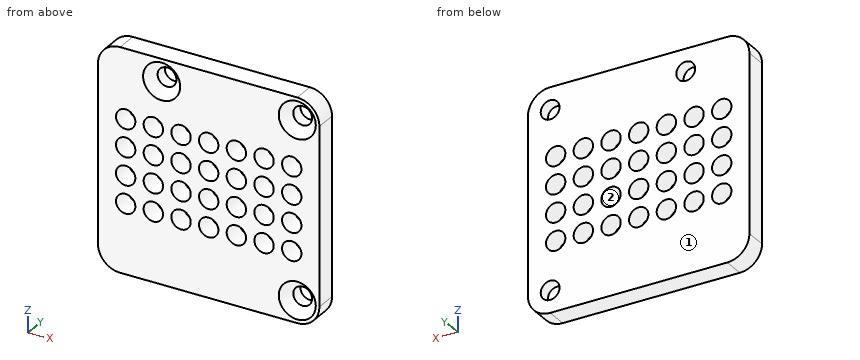
```python
from build123d import *

# Parameters (mm, degrees)
SKETCH1_R                                           = 1.6
BOSS_EXTRUDE1_DEPTH                                 = 3.85
CSK_FOR_M3_COUNTERSUNK_FLAT_HEAD_SCREW1_D           = 3.4
CSK_FOR_M3_COUNTERSUNK_FLAT_HEAD_SCREW1_CSINK_D     = 6.7
CSK_FOR_M3_COUNTERSUNK_FLAT_HEAD_SCREW1_CSINK_ANGLE = 90
SKETCH4_R                                           = 1.75
CUT_EXTRUDE1_DEPTH                                  = 12.5


with BuildPart() as part:
    # Sketch1 → Boss-Extrude1 (new body)
    with BuildSketch(Plane(origin=(0, 0, 0), x_dir=(1, 0, 0), z_dir=(0, 1, 0))):
        with BuildLine():
            Line((4, 0), (36, 0))
            ThreePointArc((36, 0), (38.828427125, 1.171572875), (40, 4))
            Line((40, 4), (40, 36))
            ThreePointArc((40, 36), (38.828427125, 38.828427125), (36, 40))
            Line((36, 40), (4, 40))
            ThreePointArc((4, 40), (1.171572875, 38.828427125), (0, 36))
            Line((0, 36), (0, 4))
            ThreePointArc((0, 4), (1.171572875, 1.171572875), (4, 0))
        make_face()
        with Locations(Location((11.5, 4, 0), (0, 0, 90))):
            Circle(SKETCH1_R, mode=Mode.SUBTRACT)
        with Locations(Location((36, 4, 0), (0, 0, 90))):
            Circle(SKETCH1_R, mode=Mode.SUBTRACT)
        with Locations(Location((36, 36, 0), (0, 0, 90))):
            Circle(SKETCH1_R, mode=Mode.SUBTRACT)
    extrude(amount=BOSS_EXTRUDE1_DEPTH)

    # CSK for M3 Countersunk Flat Head Screw1 (through all)
    with Locations(Plane(origin=(0, 0, 0), x_dir=(-1, 0, 0), z_dir=(0, -1, 0))):
        with Locations((-11.5, 4), (-36, 4), (-36, 36)):
            CounterSinkHole(CSK_FOR_M3_COUNTERSUNK_FLAT_HEAD_SCREW1_D / 2, CSK_FOR_M3_COUNTERSUNK_FLAT_HEAD_SCREW1_CSINK_D / 2, counter_sink_angle=CSK_FOR_M3_COUNTERSUNK_FLAT_HEAD_SCREW1_CSINK_ANGLE)

    # Sketch4 → Cut-Extrude1 (cut)
    with BuildSketch(Plane(origin=(0, 3.85, 0), x_dir=(1, 0, 0), z_dir=(0, 1, 0))):
        with Locations(Location((5, 22.5, 0), (0, 0, 270))):
            Circle(SKETCH4_R)
        with Locations(Location((10, 22.5, 0), (0, 0, 270))):
            Circle(SKETCH4_R)
        with Locations(Location((5, 17.5, 0), (0, 0, 270))):
            Circle(SKETCH4_R)
        with Locations(Location((10, 17.5, 0), (0, 0, 270))):
            Circle(SKETCH4_R)
        with Locations(Location((30, 17.5, 0), (0, 0, 90))):
            Circle(SKETCH4_R)
        with Locations(Location((35, 17.5, 0), (0, 0, 90))):
            Circle(SKETCH4_R)
        with Locations(Location((30, 22.5, 0), (0, 0, 90))):
            Circle(SKETCH4_R)
        with Locations(Location((35, 22.5, 0), (0, 0, 90))):
            Circle(SKETCH4_R)
        with Locations(Location((15, 22.5, 0), (0, 0, 270))):
            Circle(SKETCH4_R)
        with Locations(Location((15, 17.5, 0), (0, 0, 270))):
            Circle(SKETCH4_R)
        with Locations(Location((20, 22.5, 0), (0, 0, 270))):
            Circle(SKETCH4_R)
        with Locations(Location((20, 17.5, 0), (0, 0, 270))):
            Circle(SKETCH4_R)
        with Locations(Location((25, 22.5, 0), (0, 0, 270))):
            Circle(SKETCH4_R)
        with Locations(Location((25, 17.5, 0), (0, 0, 270))):
            Circle(SKETCH4_R)
        with Locations(Location((5, 27.5, 0), (0, 0, 270))):
            Circle(SKETCH4_R)
        with Locations(Location((10, 27.5, 0), (0, 0, 270))):
            Circle(SKETCH4_R)
        with Locations(Location((30, 27.5, 0), (0, 0, 90))):
            Circle(SKETCH4_R)
        with Locations(Location((35, 27.5, 0), (0, 0, 90))):
            Circle(SKETCH4_R)
        with Locations(Location((15, 27.5, 0), (0, 0, 270))):
            Circle(SKETCH4_R)
        with Locations(Location((20, 27.5, 0), (0, 0, 270))):
            Circle(SKETCH4_R)
        with Locations(Location((25, 27.5, 0), (0, 0, 270))):
            Circle(SKETCH4_R)
        with Locations(Location((5, 12.5, 0), (0, 0, 270))):
            Circle(SKETCH4_R)
        with Locations(Location((10, 12.5, 0), (0, 0, 270))):
            Circle(SKETCH4_R)
        with Locations(Location((30, 12.5, 0), (0, 0, 90))):
            Circle(SKETCH4_R)
        with Locations(Location((35, 12.5, 0), (0, 0, 90))):
            Circle(SKETCH4_R)
        with Locations(Location((15, 12.5, 0), (0, 0, 270))):
            Circle(SKETCH4_R)
        with Locations(Location((20, 12.5, 0), (0, 0, 270))):
            Circle(SKETCH4_R)
        with Locations(Location((25, 12.5, 0), (0, 0, 270))):
            Circle(SKETCH4_R)
    extrude(amount=-CUT_EXTRUDE1_DEPTH, mode=Mode.SUBTRACT)


solid = part.part
```
Build history of the part. All positions in model axes, mm. Face numbers are marked on the shaded views. Give positions to 0.01 mm unless a question says otherwise; leave off trailing zeros. Order: outer loops, then holes, each group sorted by start corner. A loop starts at its lowest first (then second) coordinate and runs counter-clockwise, first axis right, second up. Notation, with made-up numbers: M 60.5,46.25 L 69.5,46.25 A20 cw 69.5,53.25 Z; hole C 3.25,47 d6. An arc over 180 degrees is marked long. Return JSON: item names as keys, results as strings.
Q1. Band-saw the part on A-A (z = -17.5). Count the separate pieces of the cut face and the enclosed holes in it, then the cut area to 3 significant figures.
Answer list:
{"separate pieces": "8", "enclosed holes": "0", "area": "59.7 mm^2"}
Q2. Wall check: probe 1 along Z at (x, y) = (4, 2.55); probe 2 along Z at (x, y) = (30, 1.85); probe 3 along X at (y, z) = (2.65, -36). Give the ranges that are in metal, low to high. Write a range as from..to.
Answer list:
{"probe 1": "z = -40..-28.94, -26.06..-23.94, -21.06..-18.94, -16.06..-13.94, -11.06..0", "probe 2": "z = -40..-29.25, -25.75..-24.25, -20.75..-19.25, -15.75..-14.25, -10.75..0", "probe 3": "x = 0..34.3, 37.7..40"}
Q3. Band-saw the part on D-D (x = 26). Give the cut face in (y, z), then the cut area to 3 significant figures.
Answer list:
{"outline": "M 0,-40 L 3.85,-40 L 3.85,-28.94 L 0,-28.94 Z; M 0,-26.06 L 3.85,-26.06 L 3.85,-23.94 L 0,-23.94 Z; M 0,-21.06 L 3.85,-21.06 L 3.85,-18.94 L 0,-18.94 Z; M 0,-16.06 L 3.85,-16.06 L 3.85,-13.94 L 0,-13.94 Z; M 0,-11.06 L 3.85,-11.06 L 3.85,0 L 0,0 Z", "area": "110 mm^2"}
Q4. Two-plate mould, pull along Z, no slides. Class the marked faces 1 and 2: pulls with the +Z half, pulls with the -Z half, needs draft (parallel to the pull), parting line crosses it, or undercut.
Answer list:
{"face 1": "needs draft", "face 2": "undercut"}
Q5. Band-saw the part on B-B (x = 15.5). Give the cut face in (y, z), then the cut area to 3 significant figures.
Answer list:
{"outline": "M 0,-40 L 3.85,-40 L 3.85,-29.18 L 0,-29.18 Z; M 0,-25.82 L 3.85,-25.82 L 3.85,-24.18 L 0,-24.18 Z; M 0,-20.82 L 3.85,-20.82 L 3.85,-19.18 L 0,-19.18 Z; M 0,-15.82 L 3.85,-15.82 L 3.85,-14.18 L 0,-14.18 Z; M 0,-10.82 L 3.85,-10.82 L 3.85,0 L 0,0 Z", "area": "102 mm^2"}
Q6. Flat gauge pin, fed straight in: pin 1 (3 mm diameter, centred on x = 20, z = -22.5, fed in from -Y). Where does the tip first touch, or does it go through?
Answer list:
{"pin 1": "passes through"}
